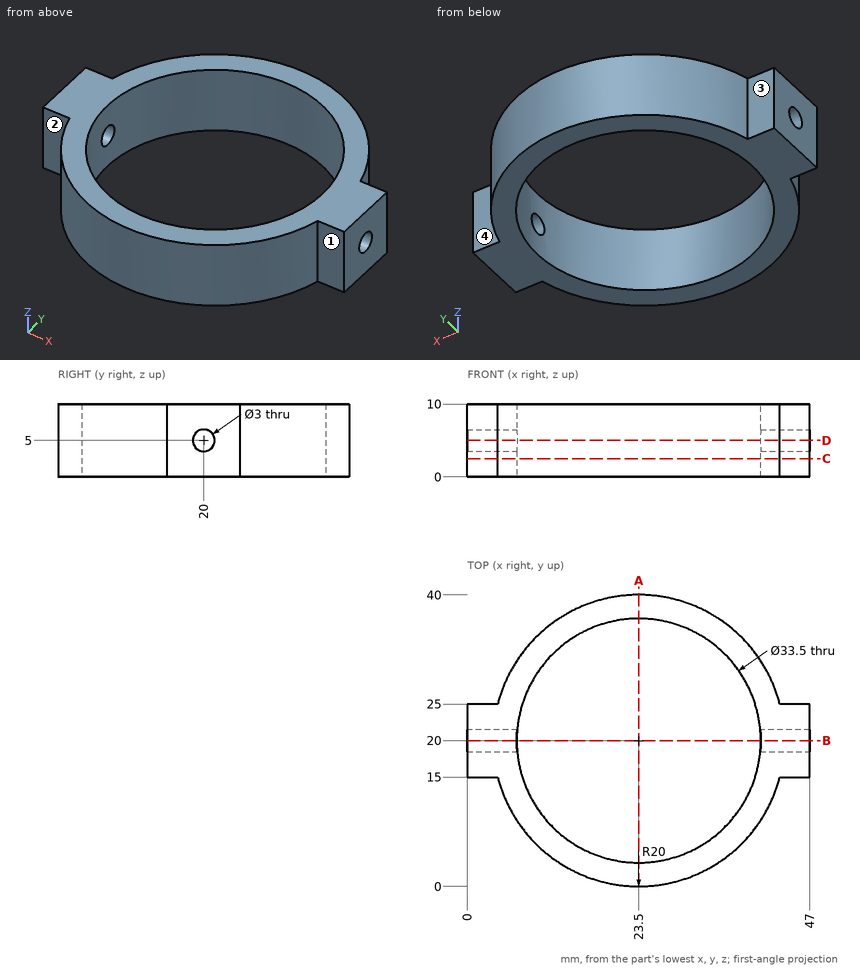
Geometry check sheet. Reference: drawing and pictorial views, mm from the part's lowest x, y, z. A direction names the side the tool comes from. Give positions to 0.01 mm unless a question says otherwise; leave off trailing zeros. Write each loop counter-clockwise with the first axis right and the second up, starting at its lowest first coordinate (ties: lowest second). Pieces come first, ordered by that corner, then holes. Notation, with made-up numbers: (-4, 74.25) - (4, 74.25) arc R29 ccw to (4, 97.25) - close; hole circle Ø2 at (46, 25.25). An arc over 180 degrees is marked (long way). Put each result on its own line as item: value.
Q1. Scan lines: probe 1 along X at (y, z) = (20, 3); probe 2 along Z at (x, y) = (45.25, 20); probe 3 along Y at (x, z) = (23, 7.75). Record each from-to range of solid material in increasing order. Write a range as from..to.
Result:
probe 1: 0..6.75, 40.25..47
probe 2: 0..3.5, 6.5..10
probe 3: 0.01..3.26, 36.74..39.99
Q2. Depth check by flat-ended pin: P1, Ø3.5, axis at x = 45.5, z = 5.5, coming from the -Y side; P2, Ø2, axis at x = 3, z = 7.5, coming from the +Y side. Enter the tip coordinate at first touch or a pass-through.
Result:
P1: y = 15
P2: y = 25
Q3. Section check B-B on y = 20. Record the cut outline in (x, z).
Result:
outline: (0, 0) - (6.75, 0) - (6.75, 3.5) - (0, 3.5) - close; (0, 6.5) - (6.75, 6.5) - (6.75, 10) - (0, 10) - close; (40.25, 0) - (47, 0) - (47, 3.5) - (40.25, 3.5) - close; (40.25, 6.5) - (47, 6.5) - (47, 10) - (40.25, 10) - close
Q4. Set-up check for the marked faces 1, 2, 3 and 4: record each of +Z, -Z, +X, -X, +Y, -Y from which the full face is reachable in a straight line by a thin tool's end or side.
Result:
face 1: +Z, -Z, +X, -Y
face 2: +Z, -Z, -X, -Y
face 3: +Z, -Z, -X, +Y
face 4: +Z, -Z, +X, +Y
Q5. Section check D-D on z = 5. Record the cut outline in (x, y).
Result:
outline: (0, 15) - (4.14, 15) arc R20 ccw to (42.86, 15) - (47, 15) - (47, 18.5) - (40.18, 18.5) arc R16.75 cw to (6.82, 18.5) - (0, 18.5) - close; (0, 21.5) - (6.82, 21.5) arc R16.75 cw to (40.18, 21.5) - (47, 21.5) - (47, 25) - (42.86, 25) arc R20 ccw to (4.14, 25) - (0, 25) - close
Q6. Section check A-A on x = 23.5. Record the cut outline in (y, z), and give its area (3 significant figures).
Result:
outline: (0, 0) - (3.25, 0) - (3.25, 10) - (0, 10) - close; (36.75, 0) - (40, 0) - (40, 10) - (36.75, 10) - close
area: 65.0 mm2
Q7. Section check C-C on z = 2.5. Record the cut outline in (x, y), and give its area (3 significant figures).
Result:
outline: (0, 15) - (4.14, 15) arc R20 ccw to (42.86, 15) - (47, 15) - (47, 25) - (42.86, 25) arc R20 ccw to (4.14, 25) - (0, 25) - close; hole circle Ø33.5 at (23.5, 20)
area: 449 mm2
